```python
from build123d import *

# Parameters (mm, degrees)
F1_R     = 1.5494
F2_DEPTH = 3.9878


with BuildPart() as f2:
    # F1 (on Right) → F2 (new body)
    with BuildSketch(Plane.YZ):
        with BuildLine():
            ThreePointArc((8.272591, 23.638659), (0, 25.0444), (-8.272591, 23.638659))
            Line((-8.272591, 23.638659), (-6.409999, 18.316365))
            ThreePointArc((-6.409999, 18.316365), (0, 19.4056), (6.409999, 18.316365))
            Line((6.409999, 18.316365), (8.272591, 23.638659))
        make_face()
        with Locations((-4.620837, 21.73933)):
            Circle(F1_R, mode=Mode.SUBTRACT)
        with Locations((0, 22.225)):
            Circle(F1_R, mode=Mode.SUBTRACT)
        with Locations((4.620837, 21.73933)):
            Circle(F1_R, mode=Mode.SUBTRACT)
    extrude(amount=F2_DEPTH)


solid = f2.part
```
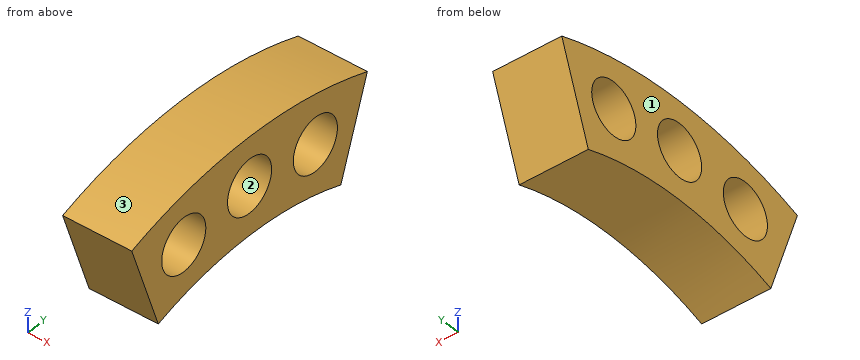
Can you work these out from the model? Positions are in its coordinate system, mm. Face numbers are marked on the shaded views. Give positions to 0.01 mm unless a question says otherwise; leave off trailing zeros. Loops run counter-clockwise (first coordinate to the right, second up) from the corner with the lowest first, then second, coordinate; pieces in that order, holes last. Notation, with made-up numbers: M 13,34.5 L 57,34.5 A19 ccw 57,65.5 Z; hole C -28.5,56.25 d6. An arc over 180 degrees is marked long. One line per question, with ' | ' between items. Start each with the question number.
Q1. If I drill on line 1 (Y direction, x = 3.6, z = 21.5); line 2 (Y direction, x = 1.85, z = 22.5); line 3 (Z direction, x = 3.25, y = -4), over which ranges is the centre line in solid material (lowest first)? Write a range as from..to.
Q2. If we section it at D-D (z = 20.5): Please give me the cut outline in (x, y).
Q3. If we section it at B-B (z = 22.5): Please give me the cut outline in (x, y).
Q4. If we section it at C-C (x = 2.25): Please give me the cut outline in (y, z) (3 decimals), plus the area to 3 significant figures.
Q5. If we mould it in two halves opening along Z, with no side actions, what happens to the marked faces 1, 2 and 3? For each: +Z half, -Z half, draft (parallel to the pull), parting line (faces both ways), or undercut.
Q6. If we section it at A-A (y = 0): Please give me the cut outline in (x, z).
Q7. For pin 1 Ø2 at (x, z) = (3.5, 20.5) entering from -Y, with a flat end and sliding along its axis, tell me the tip position at first contact or that it passes through.
Computed:
1) line 1: y = -7.52..-6.15, -3.09..-1.37, 1.37..3.09, 6.15..7.52 | line 2: y = -7.87..-5.97, -3.27..-1.52, 1.52..3.27, 5.97..7.87 | line 3: z = 18.99..20.32, 23.16..24.72
2) outline: M 0,-7.17 L 3.99,-7.17 L 3.99,-5.55 L 0,-5.55 Z; M 0,-3.69 L 3.99,-3.69 L 3.99,3.69 L 0,3.69 Z; M 0,5.55 L 3.99,5.55 L 3.99,7.17 L 0,7.17 Z
3) outline: M 0,-7.87 L 3.99,-7.87 L 3.99,-5.97 L 0,-5.97 Z; M 0,-3.27 L 3.99,-3.27 L 3.99,-1.52 L 0,-1.52 Z; M 0,1.52 L 3.99,1.52 L 3.99,3.27 L 0,3.27 Z; M 0,5.97 L 3.99,5.97 L 3.99,7.87 L 0,7.87 Z
4) outline: M -8.273,23.639 L -6.41,18.316 A19.406 cw 6.41,18.316 L 8.273,23.639 A25.044 ccw Z; hole C -4.621,21.739 d3.099; hole C 0,22.225 d3.099; hole C 4.621,21.739 d3.099 | area: 61.8 mm²
5) face 1: draft | face 2: undercut | face 3: +Z half
6) outline: M 0,19.41 L 3.99,19.41 L 3.99,20.68 L 0,20.68 Z; M 0,23.77 L 3.99,23.77 L 3.99,25.04 L 0,25.04 Z
7) pin 1: stops at y = -7.52
